from build123d import *

# Parameters (mm, degrees)
CROQUIS1_W              = 45
CROQUIS1_H              = 75
SALIENTE_EXTRUIR1_DEPTH = 1
CROQUIS2_W              = 45
CROQUIS2_H              = 11.7
SALIENTE_EXTRUIR2_DEPTH = 1.38
CROQUIS5_W              = 6.714746972
CROQUIS5_H              = 75
CORTAR_EXTRUIR2_DEPTH   = 38.3
CROQUIS7_R              = 1.75
CROQUIS7_R_2            = 1.745
SALIENTE_EXTRUIR3_DEPTH = 3
CROQUIS8_W              = 10.404122083
CROQUIS8_H              = 2.00964754
CORTAR_EXTRUIR3_DEPTH   = 40
CROQUIS9_W              = 3.216312559
CROQUIS9_H              = 9.421023217
CORTAR_EXTRUIR5_DEPTH   = 10
CROQUIS10_W             = 3.147375437
CROQUIS10_H             = 27.45813743
CROQUIS10_W_2           = 3.03884525
SALIENTE_EXTRUIR4_DEPTH = 7
CROQUIS11_W             = 24.765018181
CROQUIS11_H             = 4.681943735
CORTAR_EXTRUIR6_DEPTH   = 47
SALIENTE_EXTRUIR5_DEPTH = 3
CROQUIS13_W             = 10.418820836
CROQUIS13_H             = 2.453250219
CORTAR_EXTRUIR7_DEPTH   = 43


with BuildPart() as part:
    # Croquis1 → Saliente-Extruir1 (new body)
    with BuildSketch(Plane(origin=(0, 0, 0), x_dir=(1, 0, 0), z_dir=(0, 1, 0))):
        Rectangle(CROQUIS1_W, CROQUIS1_H)
    extrude(amount=SALIENTE_EXTRUIR1_DEPTH)

    # Croquis2 → Saliente-Extruir2 (add)
    with BuildSketch(Plane(origin=(0, 1, 0), x_dir=(1, 0, 0), z_dir=(0, 1, 0))):
        with Locations((0, 1.05)):
            Rectangle(CROQUIS2_W, CROQUIS2_H)
    extrude(amount=SALIENTE_EXTRUIR2_DEPTH)

    # Croquis5 → Cortar-Extruir2 (cut)
    with BuildSketch(Plane.XZ):
        with Locations((19.142626514, 0)):
            Rectangle(CROQUIS5_W, CROQUIS5_H)
    extrude(amount=-CORTAR_EXTRUIR2_DEPTH, mode=Mode.SUBTRACT)

    # Croquis7 → Saliente-Extruir3 (add)
    with BuildSketch(Plane(origin=(0, 1, 0), x_dir=(1, 0, 0), z_dir=(0, 1, 0))):
        with Locations((-3.357373486, 34.85)):
            Circle(CROQUIS7_R)
        with Locations((-3.357373486, -34.85)):
            Circle(CROQUIS7_R_2)
    extrude(amount=SALIENTE_EXTRUIR3_DEPTH)

    # Croquis8 → Cortar-Extruir3 (cut)
    with BuildSketch(Plane.ZY.offset(22.5)):
        with Locations((-1.128567076, 1.00482377)):
            Rectangle(CROQUIS8_W, CROQUIS8_H)
    extrude(amount=-CORTAR_EXTRUIR3_DEPTH, mode=Mode.SUBTRACT)

    # Croquis9 → Cortar-Extruir5 (cut)
    with BuildSketch(Plane.XZ.offset(-2.00964754)):
        with Locations((12.147096749, -1.030456008)):
            Rectangle(CROQUIS9_W, CROQUIS9_H)
    extrude(amount=-CORTAR_EXTRUIR5_DEPTH, mode=Mode.SUBTRACT)

    # Croquis10 → Saliente-Extruir4 (add)
    with BuildSketch(Plane.XZ):
        with Locations((12.079419824, -22.642531368)):
            Rectangle(CROQUIS10_W, CROQUIS10_H)
        with Locations((-19.448599637, -22.642531368)):
            Rectangle(CROQUIS10_W_2, CROQUIS10_H)
    extrude(amount=SALIENTE_EXTRUIR4_DEPTH)

    # Croquis11 → Cortar-Extruir6 (cut)
    with BuildSketch(Plane(origin=(13.653107542, 0, 0), x_dir=(0, 0, -1), z_dir=(1, 0, 0))):
        with Locations((22.608859882, -3.539167372)):
            Rectangle(CROQUIS11_W, CROQUIS11_H)
    extrude(amount=-CORTAR_EXTRUIR6_DEPTH, mode=Mode.SUBTRACT)

    # Croquis12 → Saliente-Extruir5 (add)
    with BuildSketch(Plane(origin=(0, 2.38, 0), x_dir=(1, 0, 0), z_dir=(0, 1, 0))):
        Polygon((10.521558479, 6.9), (-22.5, 6.9), (-22.5, -4.8), (10.521558479, -4.8), (10.521558479, 5.740967616), align=None)
        Polygon((13.755253028, 6.9), (10.521558479, 6.9), (10.521558479, 5.740967616), (10.538940469, 5.740967616), (13.755253028, 5.740967616), align=None)
        Polygon((15.785253028, 6.9), (13.792175248, 6.9), (13.792175248, -3.680055601), (13.792175248, -4.8), (15.785253028, -4.8), align=None)
        Polygon((10.538940469, -3.680055601), (10.538940469, -4.8), (13.792175248, -4.8), (13.792175248, -3.680055601), (13.755253028, -3.680055601), align=None)
    extrude(amount=SALIENTE_EXTRUIR5_DEPTH)

    # Croquis13 → Cortar-Extruir7 (cut)
    with BuildSketch(Plane(origin=(15.785253028, 0, 0), x_dir=(0, 0, -1), z_dir=(1, 0, 0))):
        with Locations((1.143850221, 3.23627265)):
            Rectangle(CROQUIS13_W, CROQUIS13_H)
    extrude(amount=-CORTAR_EXTRUIR7_DEPTH, mode=Mode.SUBTRACT)


solid = part.part
Could you check a few things on this model? Use its own coordinates, in mm. A direction names the side the tool comes from. Coordinates: 2 decimals unless noted, no trailing zeros. Loops run counter-clockwise (first coordinate to the right, second up) from the corner with the lowest first, then second, coordinate; pieces in that order, holes last.
1. I need wall thicknesses on L1, parallel to Z at x = 7, y = 3.5; L2, parallel to Z at x = -12, y = 2; L3, parallel to Y at x = 11, z = -11. Which ranges of each line are inside material? Lowest first, please.
2. Imagine slicing it at D-D (z = 8). Please give me the cut outline in (x, y), and give its area (3 significant figures).
3. We'd pull the mould along Z, two halves only. Please class faces 6 (the face through (12, -5.88, -22)), 7 (the face through (14, 5.38, 0)), 8 (the face through (12, -3, -8.913)), 9 (the face through (12, -4, -10.226)): released by +Z, released by -Z, zero draft, split by the parting line, or undercut.
4. For P1, Ø3, axis at x = -10, z = 7, coming from the +Y side; P2, Ø2, axis at x = 3.5, y = 2.5, coming from the -Z side; P3, Ø4, axis at x = -4, z = -35, coming from the +Y side; P4, Ø1, axis at y = -2, z = -13, coming from the +X side, each with a flat end and sliding along its axis, tell me the tip position at first contact or that it passes through.
5. Imagine slicing it at A-A (y = -4.75). Please give me the cut outline in (x, z).
6. Imagine slicing it at B-B (z = 34.85). Please give me the cut outline in (x, y).
7. For faces 1 (the face through (-4, 1, -6.331)), 2 (the face through (13.653, -1, -26)), 3 (the face through (-19, -4, -10.226)), 4 (the face through (-19, -3, -8.913)), 5 (the face through (12, -3, -36.372)), which set-ups out of +Z, -Z, +X, -X, +Y, -Y let a thin tool reach every point of the face, with its end or its side?
Computed values:
1. L1: z = -6.9 to -6.35, 4.07 to 4.8
1. L2: z = -6.9 to -6.33, 4.07 to 4.8
1. L3: y = -7 to -5.88, -1.2 to 1
2. outline: (-22.5, 0) - (15.79, 0) - (15.79, 1) - (-22.5, 1) - close
2. area: 38.3 mm2
3. face 6: undercut
3. face 7: zero draft
3. face 8: released by +Z
3. face 9: undercut
4. P1: stops at y = 1
4. P2: stops at z = -6.9
4. P3: stops at y = 4
4. P4: passes through
5. outline: (-20.97, -36.37) - (-17.93, -36.37) - (-17.93, -34.99) - (-20.97, -34.99) - close; (-20.97, -10.23) - (-17.93, -10.23) - (-17.93, -8.91) - (-20.97, -8.91) - close; (10.51, -36.37) - (13.65, -36.37) - (13.65, -34.99) - (10.51, -34.99) - close; (10.51, -10.23) - (13.65, -10.23) - (13.65, -8.91) - (10.51, -8.91) - close
6. outline: (-22.5, 0) - (15.79, 0) - (15.79, 1) - (-1.61, 1) - (-1.61, 4) - (-5.1, 4) - (-5.1, 1) - (-22.5, 1) - close
7. face 1: +X, -X, -Y
7. face 2: +Z, -Z, +X, -Y
7. face 3: +X, -X
7. face 4: +Z, +X, -X, -Y
7. face 5: -Z, +X, -X, -Y
